from build123d import *

# Parameters (mm, degrees)
SKETCH1_R           = 7.5
SKETCH1_R_2         = 5
BOSS_EXTRUDE1_DEPTH = 2
BOSS_EXTRUDE2_DEPTH = 2
FILLET1_R           = 10
SKETCH3_R           = 6.8
CUT_EXTRUDE1_DEPTH  = 10
SKETCH4_R           = 1.5
CUT_EXTRUDE2_DEPTH  = 10
SKETCH5_R           = 1.5
CUT_EXTRUDE3_DEPTH  = 10
SKETCH6_R           = 1.75
CUT_EXTRUDE4_DEPTH  = 179.433043373


with BuildPart() as part:
    # Sketch1 → Boss-Extrude1 (new body)
    with BuildSketch(Plane(origin=(0, 0, 0), x_dir=(1, 0, 0), z_dir=(0, 1, 0))):
        Polygon((0, 76.188021535), (-65.980762114, -38.094010768), (65.980762114, -38.094010768), align=None)
        with Locations(Location((0, 46.188021535, 0), (0, 0, 270))):
            Circle(SKETCH1_R, mode=Mode.SUBTRACT)
        with Locations(Location((-40, -23.094010768, 0), (0, 0, 270))):
            Circle(SKETCH1_R, mode=Mode.SUBTRACT)
        with Locations(Location((40, -23.094010768, 0), (0, 0, 270))):
            Circle(SKETCH1_R, mode=Mode.SUBTRACT)
        with Locations(Location((0, 0, 0), (0, 0, 270))):
            Circle(SKETCH1_R_2, mode=Mode.SUBTRACT)
    extrude(amount=BOSS_EXTRUDE1_DEPTH)

    # Sketch2 → Boss-Extrude2 (add)
    with BuildSketch(Plane(origin=(0, 2, 0), x_dir=(1, 0, 0), z_dir=(0, 1, 0))):
        Polygon((43.490381057, 0.860471904), (22.490381057, 37.233538863), (132.394191624, 100.686533479), (153.394191624, 64.313466521), align=None)
    extrude(amount=-BOSS_EXTRUDE2_DEPTH)

    # Fillet1
    fillet1_edges = [part.edges().sort_by_distance(p)[0] for p in [
        (153.394191624, 1, -64.313466521),
        (43.490381057, 1, -0.860471904),
        (22.490381057, 1, -37.233538863),
        (132.394191624, 1, -100.686533479),
        (65.980762114, 1, 38.094010768),
        (-65.980762114, 1, 38.094010768),
        (0, 1, -76.188021535),
    ]]
    fillet(fillet1_edges, radius=FILLET1_R)

    # Sketch3 → Cut-Extrude1 (cut)
    with BuildSketch(Plane(origin=(0, 2, 0), x_dir=(1, 0, 0), z_dir=(0, 1, 0))):
        with Locations(Location((129.903810568, 75, 0), (0, 0, 270))):
            Circle(SKETCH3_R)
    extrude(amount=-CUT_EXTRUDE1_DEPTH, mode=Mode.SUBTRACT)

    # Sketch4 → Cut-Extrude2 (cut)
    with BuildSketch(Plane(origin=(0, 2, 0), x_dir=(1, 0, 0), z_dir=(0, 1, 0))):
        with Locations(Location((133.564064606, 88.660254038, 0), (0, 0, 270))):
            Circle(SKETCH4_R)
        with Locations(Location((116.24355653, 78.660254038, 0), (0, 0, 270))):
            Circle(SKETCH4_R)
        with Locations(Location((126.24355653, 61.339745962, 0), (0, 0, 270))):
            Circle(SKETCH4_R)
        with Locations(Location((143.564064606, 71.339745962, 0), (0, 0, 270))):
            Circle(SKETCH4_R)
    extrude(amount=-CUT_EXTRUDE2_DEPTH, mode=Mode.SUBTRACT)

    # Sketch5 → Cut-Extrude3 (cut)
    with BuildSketch(Plane(origin=(0, 2, 0), x_dir=(1, 0, 0), z_dir=(0, 1, 0))):
        with Locations(Location((96.173048454, 73.423393759, 0), (0, 0, 270))):
            Circle(SKETCH5_R)
        with Locations(Location((57.201905284, 50.923393759, 0), (0, 0, 270))):
            Circle(SKETCH5_R)
        with Locations(Location((111.673048454, 46.576606241, 0), (0, 0, 270))):
            Circle(SKETCH5_R)
        with Locations(Location((72.701905284, 24.076606241, 0), (0, 0, 270))):
            Circle(SKETCH5_R)
    extrude(amount=-CUT_EXTRUDE3_DEPTH, mode=Mode.SUBTRACT)

    # Sketch6 → Cut-Extrude4 (cut, through all)
    with BuildSketch(Plane(origin=(0, 2, 0), x_dir=(1, 0, 0), z_dir=(0, 1, 0))):
        with Locations(Location((0, 8, 0), (0, 0, 270))):
            Circle(SKETCH6_R)
        with Locations(Location((8, 0, 0), (0, 0, 270))):
            Circle(SKETCH6_R)
        with Locations(Location((0, -8, 0), (0, 0, 270))):
            Circle(SKETCH6_R)
        with Locations(Location((-8, 0, 0), (0, 0, 270))):
            Circle(SKETCH6_R)
    extrude(amount=-CUT_EXTRUDE4_DEPTH, mode=Mode.SUBTRACT)


solid = part.part
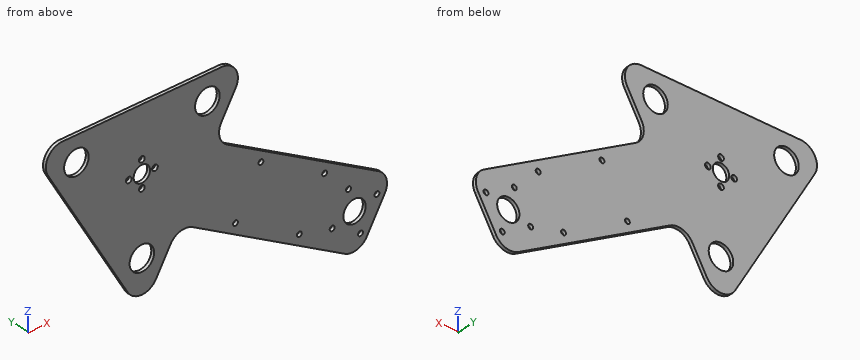
Geometry: final body of the model. Coordinates: model frame, mm. Give positions to 0.01 mm unless a question says otherwise; leave off trailing zeros. Loops run counter-clockwise (first coordinate to the right, second up) from the corner with the lowest first, then second, coordinate; pieces in that order, holes last. Notation, with made-up numbers: (58.5, 62.5) - (116.5, 62.5) arc R6 cw to (116.5, 70.5) - close; hole circle Ø7 at (25, 7.25). An arc over 180 degrees is marked (long way). Answer as CSV lines item,"result". Start each with the question number.
1. Ray query, L1, parallel to X at y = 0.6, z = -52; L2, parallel to Z at x = 3, y = 1.75; L3, parallel to Z at x = 2.5, y = 1.7. Return the intervals inside material, ascending.
2. Section C-C, the plane y = 0.7. Give the number of separate pieces and of enclosed holes in the cut face, plus the area to 3 significant figures.
3. Section D-D, the plane x = 40. Return loops of the section in (y, z).
4. Section B-B, the plane z = 21. Return loops of the section in (x, y).
5. Section A-A, the plane x = -40. Return loops of the section in (y, z), plus the area to 3 significant figures.
Answers:
1,L1,"x = -13.96 to -4.74, 4.74 to 13.96, 48.07 to 56.16, 58.25 to 132.07"
1,L2,"z = -65.73 to -53.06, -39.31 to -4, 4 to 38.09"
1,L3,"z = -65.87 to -53.26, -39.12 to -4.33, 4.33 to 38.09"
2,separate pieces,"1"
2,enclosed holes,"17"
2,area,"11,800 mm2"
3,outline,"(0, -47.34) - (2, -47.34) - (2, 15.59) - (0, 15.59) - close; (0, 30.59) - (2, 30.59) - (2, 38.09) - (0, 38.09) - close"
4,outline,"(-56.11, 0) - (-47.2, 0) - (-47.2, 2) - (-56.11, 2) - close; (-32.8, 0) - (32.8, 0) - (32.8, 2) - (-32.8, 2) - close; (47.2, 0) - (56.11, 0) - (56.11, 2) - (47.2, 2) - close"
5,outline,"(0, -6.91) - (2, -6.91) - (2, 15.59) - (0, 15.59) - close; (0, 30.59) - (2, 30.59) - (2, 38.09) - (0, 38.09) - close"
5,area,"60.0 mm2"
